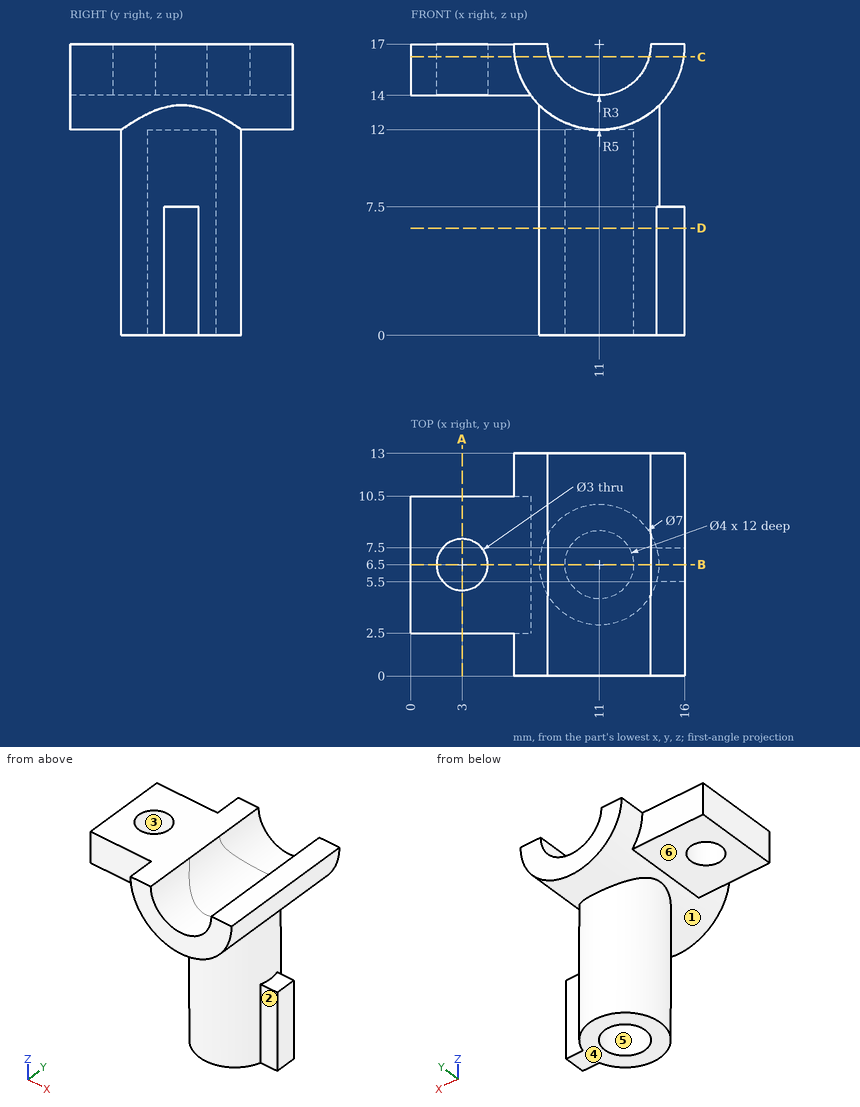
Geometry check sheet. Reference: drawing and pictorial views, mm from the part's lowest x, y, z. A direction names the side the tool comes from. Coordinates: 2 decimals unless noted, no trailing zeros. Order: outer loops, then holes, each group sorted by start corner. A loop starts at its lowest first (then second) coordinate and runs counter-clockwise, first axis right, second up. Notation, with made-up numbers: (11.5, -36.5) - (34.5, -36.5) arc R21 cw to (34.5, -19.5) - close; hole circle Ø10 at (82.5, 65.5). An arc over 180 degrees is marked (long way). Answer in a Markdown table with one row per item. Add a question column.
1) Cross-section at B-B, the plane y = 6.5. Record the cut outline in (x, z), then the cut area to 3 significant figures.
2) Material ranges on line 1 along Y through (x, z) = (3, 15); line 2 along Y through (x, z) = (11, 4); line 3 along Z through (x, y) = (5.5, 4.5), recorded low to high. Write a range as [from, to].
3) Gauge pin test, flat ends, axial feed: P1, Ø1, axis at x = 11.5, y = 6, coming from the +Z side; P2, Ø5, axis at x = 3, y = 6.5, coming from the -Z side; P3, Ø6, axis at x = 6.5, z = 3, coming from the -Y side. Record the tip position at first contact, or that the pin passes through.
4) Cross-section at A-A, the plane x = 3. Record the cut outline in (y, z), then the cut area to 3 significant figures.
5) Set-up check for the marked faces 4, 5 and 6: record each of +Z, -Z, +X, -X, +Y, -Y from which the full face is reachable in a straight line by a thin tool's end or side.
6) Cross-section at C-C, the plane z = 16.25. Record the cut outline in (x, y), then the cut area to 3 significant figures.
7) Release check for a two-part mould opening along X. For the marked faces 1, 2 and 3 record: +X half, -X half, draft (parallel to the pull), parting line (faces both ways), or undercut.
8) Cross-section at D-D, the plane z = 6.25. Record the cut outline in (x, y).
Check result:
| question | item | result |
|---|---|---|
| 1 | outline | (0, 14) - (1.5, 14) - (1.5, 17) - (0, 17) - close; (4.5, 14) - (7, 14) arc R5 ccw to (7.5, 13.43) - (7.5, 0) - (9, 0) - (9, 12) - (13, 12) - (13, 0) - (16, 0) - (16, 7.5) - (14.5, 7.5) - (14.5, 13.43) arc R5 ccw to (16, 17) - (14, 17) arc R3 cw to (8, 17) - (4.5, 17) - close |
| 1 | area | 85.5 mm² |
| 2 | line 1 | y = [2.5, 5], [8, 10.5] |
| 2 | line 2 | y = [3, 4.5], [8.5, 10] |
| 2 | line 3 | z = [14, 17] |
| 3 | P1 | stops at z = 14.17 |
| 3 | P2 | stops at z = 14 |
| 3 | P3 | stops at y = 3.34 |
| 4 | outline | (2.5, 14) - (5, 14) - (5, 17) - (2.5, 17) - close; (8, 14) - (10.5, 14) - (10.5, 17) - (8, 17) - close |
| 4 | area | 15.0 mm² |
| 5 | face 4 | -Z, +X, -X, +Y, -Y |
| 5 | face 5 | -Z |
| 5 | face 6 | -Z, -X, +Y, -Y |
| 6 | outline | (0, 2.5) - (6.06, 2.5) - (6.06, 0) - (8.1, 0) - (8.1, 13) - (6.06, 13) - (6.06, 10.5) - (0, 10.5) - close; (13.9, 0) - (15.94, 0) - (15.94, 13) - (13.9, 13) - close; hole circle Ø3 at (3, 6.5) |
| 6 | area | 94.4 mm² |
| 7 | face 1 | parting line |
| 7 | face 2 | draft |
| 7 | face 3 | undercut |
| 8 | outline | (14.35, 5.5) - (16, 5.5) - (16, 7.5) - (14.35, 7.5) arc R3.5 ccw (long way) to start; hole circle Ø4 at (11, 6.5) |
